```python
from build123d import *

# Parameters (mm, degrees)
F0_W      = 32
F0_H      = 20
F0_R      = 3.05
F1_DEPTH  = 3
F2_W      = 32
F2_H      = 20
F2_R      = 3.05
F3_DEPTH  = 4
F5_W      = 12
F5_H      = 20
F6_DEPTH  = 7.001
F4_W      = 53
F4_H      = 50
F4_R      = 1.75
F4_R_2    = 12.5
F7_DEPTH  = 7
F10_W     = 38.6691533923
F10_H     = 26.006084159
F11_DEPTH = 12.5


with BuildPart() as f1:
    # F0 (on Front) → F1 (new body)
    with BuildSketch(Plane.XZ):
        with Locations((-1.5, 0)):
            Rectangle(F0_W, F0_H)
        with Locations((4.5, 0)):
            Circle(F0_R, mode=Mode.SUBTRACT)
    extrude(amount=F1_DEPTH)

    # F2 (on face) → F3 (join)
    with BuildSketch(Plane(origin=(0, 0, 0), x_dir=(-1, 0, 0), z_dir=(0, 1, 0))):
        with Locations((1.5, 0)):
            Rectangle(F2_W, F2_H)
        with Locations((-4.5, 0)):
            Circle(F2_R, mode=Mode.SUBTRACT)
    extrude(amount=F3_DEPTH)

    # F5 (on face) → F6 (cut, through all)
    with BuildSketch(Plane(origin=(0, 4, 0), x_dir=(-1, 0, 0), z_dir=(0, 1, 0))):
        with Locations((11.5, 0)):
            Rectangle(F5_W, F5_H)
    extrude(amount=-F6_DEPTH, mode=Mode.SUBTRACT)

    # F4 (on face) → F7 (join)
    with BuildSketch(Plane(origin=(0, 4, 0), x_dir=(-1, 0, 0), z_dir=(0, 1, 0))):
        with Locations((32, 0)):
            Rectangle(F4_W, F4_H)
        with Locations((16.5, -15.5)):
            Circle(F4_R, mode=Mode.SUBTRACT)
        with Locations((47.5, -15.5)):
            Circle(F4_R, mode=Mode.SUBTRACT)
        with Locations((16.5, 15.5)):
            Circle(F4_R, mode=Mode.SUBTRACT)
        with Locations((32, 0)):
            Circle(F4_R_2, mode=Mode.SUBTRACT)
        with Locations((47.5, 15.5)):
            Circle(F4_R, mode=Mode.SUBTRACT)
    extrude(amount=-F7_DEPTH)

    # F9: F1 across plane


with BuildPart() as f1_1:
    add(f1.part)
    add(f1.part.mirror(Plane.YZ.offset(-32)))

    # F10 (on Front) → F11 (cut, symmetric)
    with BuildSketch(Plane.XZ):
        with Locations((-77.8345766962, -3.0030420795)):
            Rectangle(F10_W, F10_H)
    extrude(amount=F11_DEPTH, both=True, mode=Mode.SUBTRACT)


solid = f1_1.part
```
Geometry: final body of the model. Coordinates: model frame, mm. A direction names the side the tool comes from. Round coordinates to 2 decimals unless told otherwise and drop trailing zeros. Order: outer loops, then holes, each group sorted by start corner. A loop starts at its lowest first (then second) coordinate and runs counter-clockwise, first axis right, second up. Notation, with made-up numbers: (39.25, 87) - (83.25, 87) arc R28 cw to (83.25, 112) - close; hole circle Ø7 at (5, 65.5). An arc over 180 degrees is marked (long way). Write item = value, one per line. Start each with the question number.
Q1. Pin query (flat end, axial travel): pin 1 (3.5 mm diameter, centred on x = 8, y = -1, fed in from -Z); pin 2 (3 mm diameter, centred on x = -47.5, z = 15.5, fed in from -Y); pin 3 (10 mm diameter, centred on x = 4.5, z = 0, fed in from -Y); pin 4 (2 mm diameter, centred on x = 7, y = 2, fed in from +Z). Return the tip coordinate at first contact, or that it passes through.
Q2. Access query for faces 1 (the flat face through (-21, 4, 11)), 2 (the flat face through (5, 0, 10)), 3 (the flat face through (5, 0, -10)). Directions: +Z, -Z, +X, -X, +Y, -Y. A direction counts if a zero-diameter tool reaches every point of the face in a straight line with its end or side. Return the directions, or none.
Q3. Cut plane B-B on z = -7.5. Return the cut outline in (x, y).
Q4. Cut plane C-C on y = 1.5. Return the cut outline in (x, z).
Q5. Cut plane A-A on x = -16.5. Return the cut outline in (y, z).
Q6. Pull-direction query (X, two-part tool) for faces 4 (the flat face through (-21, -3, 11)), 5 (the flat face through (-58.5, 1, 0)), 6 (the flat face through (-5.5, 1, -18)), 7 (the cylindrical face through (-16.272, 0.549, -13.765)); classes: +X half, -X half, draft (parallel to the pull), parting line (faces both ways), or undercut.
Q7. Cut plane D-D on x = -32. Return the cut outline in (y, z), and give its area (3 significant figures).
Q8. Ray query, line 1 (X direction, y = -1.2, z = 0); line 2 (X direction, y = -1.25, z = 15.5); line 3 (Z direction, x = -16.5, y = 0.5). Return the intervals inside material, ascending. Write a range as from..to.
Outcome:
q1.pin_1 = -10
q1.pin_2 = through
q1.pin_3 = -3
q1.pin_4 = 10
q2.face_1 = +Z, -Z, +X, -X, +Y
q2.face_2 = +Z, +X, +Y, -Y
q2.face_3 = -Z, +X, +Y, -Y
q3.outline = (-58.5, -3) - (-42, -3) - (-42, 4) - (-58.5, 4) - close; (-22, -3) - (14.5, -3) - (14.5, 4) - (-22, 4) - close
q4.outline = (-58.5, -25) - (-5.5, -25) - (-5.5, -10) - (14.5, -10) - (14.5, 10) - (-5.5, 10) - (-5.5, 25) - (-58.5, 25) - close; hole circle Ø3.5 at (-47.5, -15.5); hole circle Ø3.5 at (-47.5, 15.5); hole circle Ø25 at (-32, 0); hole circle Ø3.5 at (-16.5, -15.5); hole circle Ø3.5 at (-16.5, 15.5); hole circle Ø6.1 at (4.5, 0)
q5.outline = (-3, -25) - (4, -25) - (4, -17.25) - (-3, -17.25) - close; (-3, -13.75) - (4, -13.75) - (4, 13.75) - (-3, 13.75) - close; (-3, 17.25) - (4, 17.25) - (4, 25) - (-3, 25) - close
q6.face_4 = draft
q6.face_5 = -X half
q6.face_6 = +X half
q6.face_7 = undercut
q7.outline = (-3, -25) - (4, -25) - (4, -12.5) - (-3, -12.5) - close; (-3, 12.5) - (4, 12.5) - (4, 25) - (-3, 25) - close
q7.area = 175 mm^2
q8.line_1 = -58.5..-44.5, -19.5..1.45, 7.55..14.5
q8.line_2 = -58.5..-49.25, -45.75..-18.25, -14.75..-5.5
q8.line_3 = -25..-17.25, -13.75..13.75, 17.25..25
